from build123d import *

# Parameters (mm, degrees)
F0_W     = 177.8
F0_H     = 139.7
F0_W_2   = 171.45
F2_DEPTH = 6.35
F3_D     = 21.1666666667
F3_DEPTH = 12.7
F3_TIP   = 6.359108218


with BuildPart() as f2:
    # F0 (on Front) → F2 (new body)
    with BuildSketch(Plane.XZ):
        with Locations((-176.7342258394, -41.7917792348)):
            Rectangle(F0_W, F0_H)
        with Locations((1.0657741606, -41.7917792348)):
            Rectangle(F0_W, F0_H)
        with Locations((175.6907741606, -41.7917792348)):
            Rectangle(F0_W_2, F0_H)
    extrude(amount=F2_DEPTH)

    # F3
    with Locations(Plane(origin=(0, 0, 0), x_dir=(1, 0, 0), z_dir=(0, 1, 0))):
        with Locations((-227.5342258394, 3.6917792348), (-189.4342258394, 3.6917792348), (-227.5342258394, 79.8917792348), (-51.850892506, 3.6917792348), (-13.750892506, 3.6917792348), (-51.850892506, 79.8917792348), (123.8324408273, 3.6917792348), (161.9324408273, 3.6917792348), (123.8324408273, 79.8917792348), (229.6657741606, 3.6917792348)):
            Hole(F3_D / 2, depth=F3_DEPTH)
            with Locations((0, 0, -(F3_DEPTH + F3_TIP / 2))):  # 118° drill point
                Cone(0, F3_D / 2, F3_TIP, mode=Mode.SUBTRACT)


solid = f2.part
Check sheet for the modelled part. Datum: model origin and axes. Units: mm. Coordinates: 2 decimals unless noted, no trailing zeros. Write item = value, one per line. Start each with the question number.
1. Section check A-A on z = 2. Give the number of separate pieces and of enclosed holes in the cut face, then the cut area to 3 significant figures.
2. Draft check along X on faces 1 (the cylindrical face through (-237.63, -3.22, -6.87)), 2 (the flat face through (-6, -6.35, -41)). Enter one of: released by +X, released by -X, zero draft, split by the parting line, or undercut.
3. Material ranges on line 1 (Z direction, x = -228, y = -2.5); line 2 (Z direction, x = -225, y = -6); line 3 (X direction, y = -4.5, z = -84), recorded low to high.
4. Depth check by flat-ended pin: P1, Ø12.5, axis at x = -227.53, z = -3.69, coming from the +Y side; P2, Ø5, axis at x = 195.5, z = -87.5, coming from the +Y side. Enter the tip coordinate at first touch or a pass-through.
Responses:
q1.separate_pieces = 8
q1.enclosed_holes = 0
q1.area = 2,550 mm2
q2.face_1 = undercut
q2.face_2 = zero draft
q3.line_1 = -111.64 to -90.46, -69.32 to -14.26, 6.88 to 28.06
q3.line_2 = -111.64 to -90.17, -69.62 to -13.97, 6.58 to 28.06
q3.line_3 = -265.63 to -237.29, -217.78 to -61.6, -42.1 to 114.08, 133.59 to 261.42
q4.P1 = through
q4.P2 = 0
